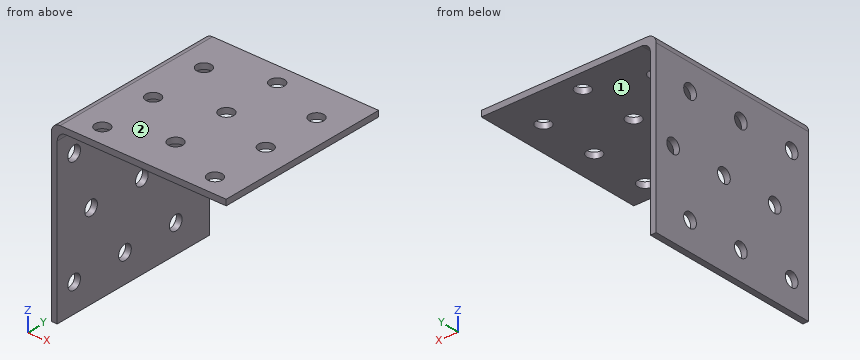
```python
from build123d import *

# Parameters (mm, degrees)
BOSS_EXTRUDE1_DEPTH = 30
SKETCH2_R           = 2.5
CUT_EXTRUDE1_DEPTH  = 10


with BuildPart() as part:
    # Sketch1 → Boss-Extrude1 (new, symmetric)
    with BuildSketch(Plane(origin=(0, 0, 0), x_dir=(1, 0, 0), z_dir=(0, 1, 0))):
        with BuildLine():
            Line((0, 3), (0, 60))
            Line((0, 60), (2, 60))
            Line((2, 60), (2, 5))
            ThreePointArc((2, 5), (2.878679656, 2.878679656), (5, 2))
            Line((5, 2), (60, 2))
            Line((60, 2), (60, 0))
            Line((60, 0), (3, 0))
            ThreePointArc((3, 0), (0.878679656, 0.878679656), (0, 3))
        make_face()
    extrude(amount=BOSS_EXTRUDE1_DEPTH, both=True)

    # Sketch2 → Cut-Extrude1 (cut)
    with BuildSketch(Plane(origin=(0, 0, -2), x_dir=(-1, 0, 0), z_dir=(0, 0, -1))):
        with Locations((-50.333333333, -23.333333333)):
            Circle(SKETCH2_R)
        with Locations((-50.333333333, -3.333333333)):
            Circle(SKETCH2_R)
        with Locations((-50.333333333, 16.666666667)):
            Circle(SKETCH2_R)
        with Locations((-31, 23.333333333)):
            Circle(SKETCH2_R)
        with Locations((-31, 3.333333333)):
            Circle(SKETCH2_R)
        with Locations((-31, -16.666666667)):
            Circle(SKETCH2_R)
        with Locations((-11.666666667, -23.333333333)):
            Circle(SKETCH2_R)
        with Locations((-11.666666667, -3.333333333)):
            Circle(SKETCH2_R)
        with Locations((-11.666666667, 16.666666667)):
            Circle(SKETCH2_R)
    cut_extrude1 = extrude(amount=-CUT_EXTRUDE1_DEPTH, mode=Mode.SUBTRACT)

    # Mirror9: Cut-Extrude1 across plane
    add(cut_extrude1.mirror(Plane(origin=(0, 0, 0), x_dir=(-0.7071067811865488, 0, 0.7071067811865462), z_dir=(0.7071067811865465, 0, 0.7071067811865487))), mode=Mode.SUBTRACT)


solid = part.part
```
CAD build for the part. Positions are in the model's coordinates, mm. Face numbers are marked on the shaded views. A direction names the side the tool comes from. Coordinates: 2 decimals unless noted, no trailing zeros. Order: outer loops, then holes, each group sorted by start corner. A loop starts at its lowest first (then second) coordinate and runs counter-clockwise, first axis right, second up. Notation, with made-up numbers: M 63.25,83 L 108.25,83 A18 ccw 108.25,89 Z; hole C -18.5,-20 d9. An arc over 180 degrees is marked long. Write each question's results on one line, items separated by ' | '. Start each with the question number.
Q1. Flat gauge pin, fed straight in: P1, Ø6.5, axis at x = 31, y = 3.33, coming from the -Z side. Where does the tip first touch, or does it go through?
Q2. Cut at D-D (x = 43). List the corners of the cut face in (y, z), then the cut area to 3 significant figures.
Q3. Which spindle directions (+Z, -Z, +X, -X, +Y, -Y) get a long thin tool onto all of the face, cutting with end or side? Do the marked faces 1 and 2. Say none if no direction does.
Q4. Cut at A-A (z = -31). List the corners of the cut face in (x, y).
Q5. Drill centre lines: probe 1 along Y at (x, z) = (31, -0.9); probe 2 along Z at (x, y) = (32.5, 6.5); probe 3 along X at (y, z) = (27, -13.5). Where is each one in solid material? Low to high. Write a range as from..to.
Q6. Cut at B-B (x = 31). List the corners of the cut face in (y, z), then the cut area to 3 significant figures.
Q7. Cut at C-C (y = 12.5). List the corners of the cut face in (x, z), then the cut area to 3 significant figures.
Found:
1) P1: z = -2
2) outline: M -30,-2 L 30,-2 L 30,0 L -30,0 Z | area: 120 mm²
3) face 1: -Z, +X, +Y, -Y | face 2: +Z, +X, -X, +Y, -Y
4) outline: M 0,-30 L 2,-30 L 2,-19.17 L 0,-19.17 Z; M 0,-14.17 L 2,-14.17 L 2,0.83 L 0,0.83 Z; M 0,5.83 L 2,5.83 L 2,20.83 L 0,20.83 Z; M 0,25.83 L 2,25.83 L 2,30 L 0,30 Z
5) probe 1: -30..-19.17, -14.17..0.83, 5.83..20.83, 25.83..30 | probe 2: -2..0 | probe 3: 0..2
6) outline: M -30,-2 L -19.17,-2 L -19.17,0 L -30,0 Z; M -14.17,-2 L 0.83,-2 L 0.83,0 L -14.17,0 Z; M 5.83,-2 L 20.83,-2 L 20.83,0 L 5.83,0 Z; M 25.83,-2 L 30,-2 L 30,0 L 25.83,0 Z | area: 90.0 mm²
7) outline: M 0,-60 L 2,-60 L 2,-5 A3 cw 5,-2 L 60,-2 L 60,0 L 3,0 A3 ccw 0,-3 Z | area: 236 mm²
